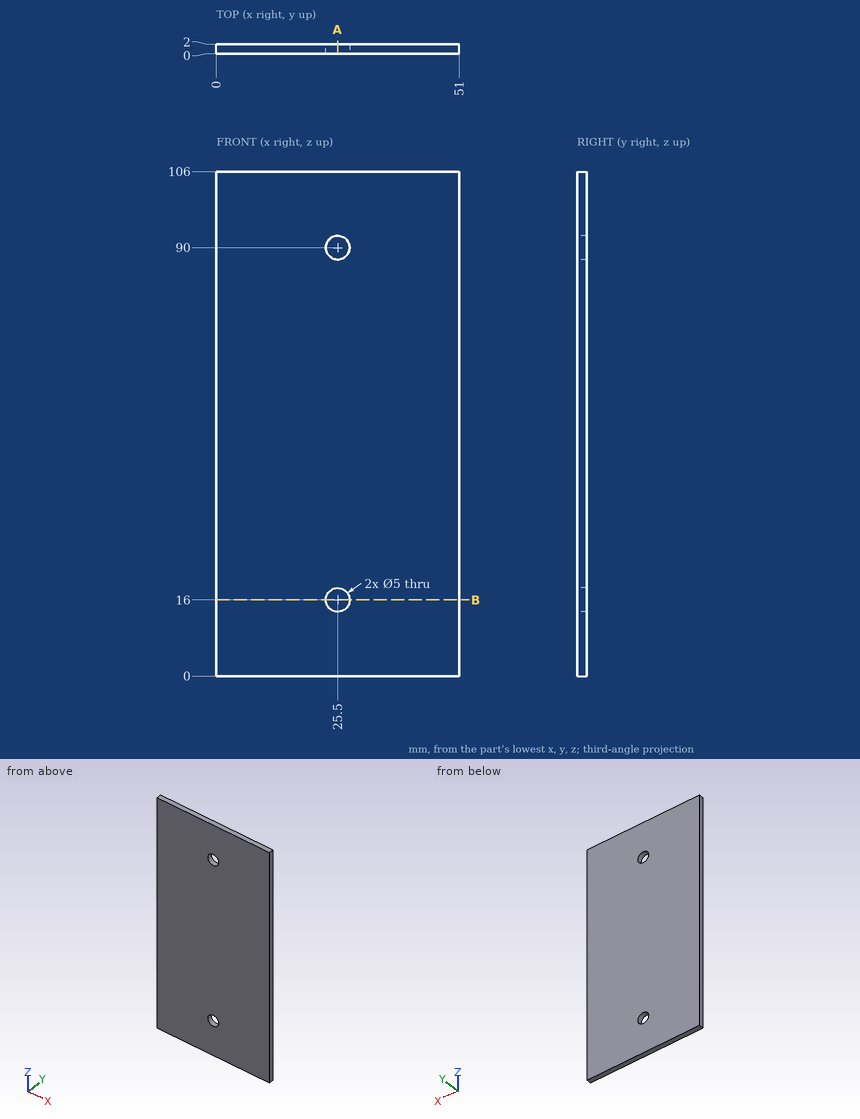
The figure shows three views and two pictorial views of one solid part (mm, origin at its lowest corner). Answer the questions. Give positions to 0.01 mm unless a question says otherwise; leave off trailing zeros. Order: outer loops, then holes, each group sorted by start corner. A loop starts at its lowest first (then second) coordinate and runs counter-clockwise, first axis right, second up. Notation, with made-up numbers: (-16, 20.25) -> (29, 20.25) arc R26 ccw to (29, 57.25) -> close; hole circle Ø5 at (39, 33). An arc over 180 degrees is marked (long way). Answer as CSV lines item,"result". Start each with the question number.
Q1. A cutting plane is placed at B-B (z = 16). Determine the outline of the cut face in (x, y), then the cut area to 3 significant figures.
Q2. A cutting plane is placed at A-A (x = 25.5). Determine the outline of the cut face in (y, z).
Q3. Find the intervals of material crossed by L1, parallel to Z at x = 25.5, y = 0.9; L2, parallel to X at y = 0.9, z = 90; L3, parallel to X at y = 0.3, z = 14, in increasing order.
Results found:
1,outline,"(0, 0) -> (23, 0) -> (23, 2) -> (0, 2) -> close; (28, 0) -> (51, 0) -> (51, 2) -> (28, 2) -> close"
1,area,"92.0 mm2"
2,outline,"(0, 0) -> (2, 0) -> (2, 13.5) -> (0, 13.5) -> close; (0, 18.5) -> (2, 18.5) -> (2, 87.5) -> (0, 87.5) -> close; (0, 92.5) -> (2, 92.5) -> (2, 106) -> (0, 106) -> close"
3,L1,"0 to 13.5, 18.5 to 87.5, 92.5 to 106"
3,L2,"0 to 23, 28 to 51"
3,L3,"0 to 24, 27 to 51"
